```python
from build123d import *

# Parameters (mm, degrees)
SKETCH1_W                     = 590.55
SKETCH1_H                     = 25.4
BOSS_EXTRUDE1_DEPTH           = 12.7
F_94_0_3_DIAMETER_HOLE1_D     = 7.62
F_94_0_3_DIAMETER_HOLE1_DEPTH = 12.7
F_94_0_3_DIAMETER_HOLE1_TIP   = 2.289278958


with BuildPart() as part:
    # Sketch1 → Boss-Extrude1 (new body)
    with BuildSketch(Plane(origin=(0, 0, 0), x_dir=(1, 0, 0), z_dir=(0, 1, 0))):
        Rectangle(SKETCH1_W, SKETCH1_H)
    extrude(amount=BOSS_EXTRUDE1_DEPTH)

    # #94 (0.3) Diameter Hole1
    with Locations(Plane(origin=(0, 12.7, 0), x_dir=(1, 0, 0), z_dir=(0, 1, 0))):
        with Locations((-269.875, 6.35), (-212.725, 6.35), (142.875, 6.35), (-155.575, 6.35), (-98.425, 6.35), (-41.275, 6.35), (15.875, 6.35), (200.025, 6.35), (257.175, 6.35)):
            Hole(F_94_0_3_DIAMETER_HOLE1_D / 2, depth=F_94_0_3_DIAMETER_HOLE1_DEPTH)
            with Locations((0, 0, -(F_94_0_3_DIAMETER_HOLE1_DEPTH + F_94_0_3_DIAMETER_HOLE1_TIP / 2))):  # 118° drill point
                Cone(0, F_94_0_3_DIAMETER_HOLE1_D / 2, F_94_0_3_DIAMETER_HOLE1_TIP, mode=Mode.SUBTRACT)


solid = part.part
```
Geometry: final body of the model. Coordinates: model frame, mm. Round coordinates to 2 decimals unless told otherwise and drop trailing zeros.
Item 1: Section query A-A (y = 7.5). Give the number of separate pieces and of enclosed holes in the cut face, plus the area to 3 significant figures.
Item 2: Material intervals for L1, parallel to Z at x = 142, y = 4; L2, parallel to Z at x = -210.5, y = 2.5, sorted ascending.
Item 3: Pin query (flat end, axial travel): P1, Ø4.5, axis at x = 15.875, z = -6.35, coming from the -Y side. Return the tip coordinate at first contact, or that it passes through.
Completed:
1. separate pieces: 1
1. enclosed holes: 9
1. area: 14,600 mm2
2. L1: z = -12.7 to -10.06, -2.64 to 12.7
2. L2: z = -12.7 to -9.44, -3.26 to 12.7
3. P1: passes through
